```python
from build123d import *

# Parameters (mm, degrees)
SKETCH_1_W               = 20
SKETCH_1_H               = 20
SKETCH_1_R               = 2
SKETCH_1_R_2             = 2.15
EXTRUDE_1_DEPTH          = 380
CUT_EXTRUDE_1_REACH      = 382.263
PATTERN_CIRCULAR_1_COUNT = 4
FILLET_1_R               = 0.3


with BuildPart() as part:
    # Sketch 1 → Extrude 1 (new body)
    with BuildSketch(Plane.XY):
        Rectangle(SKETCH_1_W, SKETCH_1_H)
        with Locations((-7, 7)):
            Circle(SKETCH_1_R, mode=Mode.SUBTRACT)
        with Locations((-7, -7)):
            Circle(SKETCH_1_R, mode=Mode.SUBTRACT)
        Circle(SKETCH_1_R_2, mode=Mode.SUBTRACT)
        with Locations((7, 7)):
            Circle(SKETCH_1_R, mode=Mode.SUBTRACT)
        with Locations((7, -7)):
            Circle(SKETCH_1_R, mode=Mode.SUBTRACT)
    extrude(amount=EXTRUDE_1_DEPTH)

    # Sketch 1_3 → Cut-Extrude 1 (cut, up to next)
    with BuildSketch(Plane.XY, mode=Mode.PRIVATE) as cut_extrude_1_sk1:
        with BuildLine():
            Line((-8.5, 2.65), (-10, 2.65))
            Line((-10, 2.65), (-10, -2.65))
            Line((-10, -2.65), (-8.5, -2.65))
            Line((-8.5, -2.65), (-8.5, -4.15))
            Line((-8.5, -4.15), (-4.503166667, -4.15))
            ThreePointArc((-4.503166667, -4.15), (-3.3, 0), (-4.503166667, 4.15))
            Line((-4.503166667, 4.15), (-8.5, 4.15))
            Line((-8.5, 4.15), (-8.5, 2.65))
        make_face()
    cut_extrude_1_tool1 = extrude(cut_extrude_1_sk1.sketch, amount=CUT_EXTRUDE_1_REACH, mode=Mode.PRIVATE) & part.part
    cut_extrude_1 = cut_extrude_1_tool1.solids().sort_by_distance((-6.606913, 0, 0))[0]
    add(cut_extrude_1, mode=Mode.SUBTRACT)

    # Pattern Circular 1: Cut-Extrude 1 ×4 about axis
    pattern_circular_1_axis = Axis((0, 0, 0), (0, 0, 1))
    for i in range(1, PATTERN_CIRCULAR_1_COUNT):
        add(cut_extrude_1.rotate(pattern_circular_1_axis, i * 360 / PATTERN_CIRCULAR_1_COUNT), mode=Mode.SUBTRACT)

    # Fillet 1
    fillet_1_edges = [part.edges().sort_by_distance(p)[0] for p in [
        (-10, -10, 190),
        (10, -10, 190),
        (10, 10, 190),
        (-10, 10, 190),
    ]]
    fillet(fillet_1_edges, radius=FILLET_1_R)


solid = part.part
```
The model under review builds one solid part; all positions refer to its coordinate system, in mm. A direction names the side the tool comes from. Coordinates: 2 decimals unless noted, no trailing zeros.
1) Machinability: for faces 1 (the face through (-3.3, -0.1, 187.3)), 2 (the face through (-10, 6, 187)), which of the approach directions +Z, -Z, +X, -X, +Y, -Y give a long, thin tool a straight path to every point of the face, cutting with its end or side? Answer none if there is none.
2) We need section A-A on z = 196. Count the separate pieces of the cut face and the enclosed holes in it, then the cut area to 3 significant figures.
3) To check wall thickness, follow probe 1 along Y at (x, z) = (7, 221.5); probe 2 along X at (y, z) = (-6.5, 116.5). State the ranges of each line that lie inside material, in increasing order.
4) The part is to be moulded in two halves that separate along X. For faces 3 (the face through (10, -6, 187)), 4 (the face through (-10, -6, 187)), 5 (the face through (0.1, -3.3, 187.3)), 6 (the face through (-2.4, 0.1, 380)), say which applies: pulls with the +X half, pulls with the -X half, needs draft (parallel to the pull), parting line crosses it, or undercut.
Answer list:
1. face 1: +Z, -Z
1. face 2: +Z, -Z, -X, +Y, -Y
2. separate pieces: 1
2. enclosed holes: 5
2. area: 144 mm2
3. probe 1: y = -10 to -9, -5 to -4.15, 4.15 to 5, 9 to 10
3. probe 2: x = -10 to -8.94, -5.06 to -4.15, 4.15 to 5.06, 8.94 to 10
4. face 3: pulls with the +X half
4. face 4: pulls with the -X half
4. face 5: undercut
4. face 6: needs draft
